For this review, take the finished solid that the model builds, in its own axes (mm). Give positions to 0.01 mm unless a question says otherwise; leave off trailing zeros. Order: outer loops, then holes, each group sorted by start corner. A loop starts at its lowest first (then second) coordinate and runs counter-clockwise, first axis right, second up. Notation, with made-up numbers: (1, 0.25) -> (31, 0.25) arc R22 ccw to (31, 31.25) -> close; hole circle Ø3 at (-28.5, 57). An arc over 180 degrees is marked (long way). Return JSON: item names as keys, results as strings. Group by question number.
1) To check wall thickness, follow line 1 along X through (y, z) = (61, 4.5); line 2 along X through (y, z) = (83.1, 0.9); line 3 along Z through (x, y) = (4.25, 79). State the ranges of each line that lie inside material, in increasing order.
2) Insertion check: P1, Ø5, axis at y = 66, z = 8.5, coming from the -X side; P2, Ø2.5, axis at x = 2, z = 4, coming from the +Y side; P3, Ø1.5, axis at x = 1.5, z = 6, coming from the +Y side. Each pin has a flat end and moves straight along its axis. Give the tip position at first contact, or say it passes through.
3) Add section D-D (y = 6). Give the boundary of the cut face in (x, z).
4) Add section A-A (y = -4.5). Give the boundary of the cut face in (x, z).
5) Add section B-B (z = 6). State how many separate pieces and enclosed holes the cut face has, then the cut area to 4 significant figures.
Autodesk Fusion 360 part; units mm, degrees
sketch "スケッチ1" plane through (0, 0, 0) normal (0, 0, 1) x (1, 0, 0)
  line L0 (1.5, 1.2) -> (3.5, 1.2)
  line L1 (3.5, 1.2) -> (3.5, 2.4)
  line L2 (3.5, 2.4) -> (1.5, 2.4)
  line L3 (1.5, 2.4) -> (1.5, 1.2)
  line L4 (1.5, 6.2) -> (3.5, 6.2)
  line L5 (3.5, 7.4) -> (1.5, 7.4)
  line L6 (3.5, 6.2) -> (3.5, 7.4)
  line L7 (1.5, 7.4) -> (1.5, 6.2)
  line L8 (1.5, 11.2) -> (3.5, 11.2)
  line L9 (3.5, 12.4) -> (1.5, 12.4)
  line L10 (3.5, 11.2) -> (3.5, 12.4)
  line L11 (1.5, 12.4) -> (1.5, 11.2)
  line L12 (1.5, 16.2) -> (3.5, 16.2)
  line L13 (3.5, 17.4) -> (1.5, 17.4)
  line L14 (3.5, 16.2) -> (3.5, 17.4)
  line L15 (1.5, 17.4) -> (1.5, 16.2)
  line L16 (1.5, 21.2) -> (3.5, 21.2)
  line L17 (3.5, 22.4) -> (1.5, 22.4)
  line L18 (3.5, 21.2) -> (3.5, 22.4)
  line L19 (1.5, 22.4) -> (1.5, 21.2)
  line L20 (1.5, 26.2) -> (3.5, 26.2)
  line L21 (3.5, 27.4) -> (1.5, 27.4)
  line L22 (3.5, 26.2) -> (3.5, 27.4)
  line L23 (1.5, 27.4) -> (1.5, 26.2)
  line L24 (1.5, 31.2) -> (3.5, 31.2)
  line L25 (3.5, 32.4) -> (1.5, 32.4)
  line L26 (3.5, 31.2) -> (3.5, 32.4)
  line L27 (1.5, 32.4) -> (1.5, 31.2)
  line L28 (1.5, 36.2) -> (3.5, 36.2)
  line L29 (3.5, 37.4) -> (1.5, 37.4)
  line L30 (3.5, 36.2) -> (3.5, 37.4)
  line L31 (1.5, 37.4) -> (1.5, 36.2)
  line L32 (1.5, 41.2) -> (3.5, 41.2)
  line L33 (3.5, 42.4) -> (1.5, 42.4)
  line L34 (3.5, 41.2) -> (3.5, 42.4)
  line L35 (1.5, 42.4) -> (1.5, 41.2)
  line L36 (1.5, 46.2) -> (3.5, 46.2)
  line L37 (3.5, 47.4) -> (1.5, 47.4)
  line L38 (3.5, 46.2) -> (3.5, 47.4)
  line L39 (1.5, 47.4) -> (1.5, 46.2)
  line L40 (1.5, 51.2) -> (3.5, 51.2)
  line L41 (3.5, 52.4) -> (1.5, 52.4)
  line L42 (3.5, 51.2) -> (3.5, 52.4)
  line L43 (1.5, 52.4) -> (1.5, 51.2)
  line L44 (1.5, 56.2) -> (3.5, 56.2)
  line L45 (3.5, 57.4) -> (1.5, 57.4)
  line L46 (3.5, 56.2) -> (3.5, 57.4)
  line L47 (1.5, 57.4) -> (1.5, 56.2)
  line L48 (1.5, 61.2) -> (3.5, 61.2)
  line L49 (3.5, 62.4) -> (1.5, 62.4)
  line L50 (3.5, 61.2) -> (3.5, 62.4)
  line L51 (1.5, 62.4) -> (1.5, 61.2)
  line L52 (1.5, 66.2) -> (3.5, 66.2)
  line L53 (3.5, 67.4) -> (1.5, 67.4)
  line L54 (3.5, 66.2) -> (3.5, 67.4)
  line L55 (1.5, 67.4) -> (1.5, 66.2)
  line L56 (1.5, 71.2) -> (3.5, 71.2)
  line L57 (3.5, 72.4) -> (1.5, 72.4)
  line L58 (3.5, 71.2) -> (3.5, 72.4)
  line L59 (1.5, 72.4) -> (1.5, 71.2)
  line L60 (1.5, 76.2) -> (3.5, 76.2)
  line L61 (3.5, 77.4) -> (1.5, 77.4)
  line L62 (3.5, 76.2) -> (3.5, 77.4)
  line L63 (1.5, 77.4) -> (1.5, 76.2)
  line L64 (0, 78.6) -> (5, 78.6)
  line L65 (5, 78.6) -> (5, 0)
  line L66 (5, 0) -> (0, 0)
  line L67 (0, 0) -> (0, 78.6)
  line L68 (6.5, -1.5) -> (-1.5, -1.5)
  line L69 (-1.5, -1.5) -> (-1.5, 80.1)
  line L70 (-1.5, 80.1) -> (6.5, 80.1)
  line L71 (6.5, 80.1) -> (6.5, -1.5)
  line L72 (0, 5.1) -> (5, 5.1)
  line L73 (5, 5.1) -> (5, 3.6)
  line L74 (5, 3.6) -> (0, 3.6)
  line L75 (0, 3.6) -> (0, 5.1)
  line L76 (5, 8.6) -> (0, 8.6)
  line L77 (0, 10.1) -> (5, 10.1)
  line L78 (5, 13.6) -> (0, 13.6)
  line L79 (0, 15.1) -> (5, 15.1)
  line L80 (5, 18.6) -> (0, 18.6)
  line L81 (0, 20.1) -> (5, 20.1)
  line L82 (5, 23.6) -> (0, 23.6)
  line L83 (0, 25.1) -> (5, 25.1)
  line L84 (5, 28.6) -> (0, 28.6)
  line L85 (0, 30.1) -> (5, 30.1)
  line L86 (5, 33.6) -> (0, 33.6)
  line L87 (0, 35.1) -> (5, 35.1)
  line L88 (5, 38.6) -> (0, 38.6)
  line L89 (0, 40.1) -> (5, 40.1)
  line L90 (5, 43.6) -> (0, 43.6)
  line L91 (0, 45.1) -> (5, 45.1)
  line L92 (5, 48.6) -> (0, 48.6)
  line L93 (0, 50.1) -> (5, 50.1)
  line L94 (5, 53.6) -> (0, 53.6)
  line L95 (0, 55.1) -> (5, 55.1)
  line L96 (5, 58.6) -> (0, 58.6)
  line L97 (0, 60.1) -> (5, 60.1)
  line L98 (5, 63.6) -> (0, 63.6)
  line L99 (0, 65.1) -> (5, 65.1)
  line L100 (5, 68.6) -> (0, 68.6)
  line L101 (0, 70.1) -> (5, 70.1)
  line L102 (5, 73.6) -> (0, 73.6)
  line L103 (0, 75.1) -> (5, 75.1)
  line L104 (-1.5, 80.1) -> (6.5, 80.1)
  line L105 (6.5, 80.1) -> (6.5, 86.1)
  line L106 (6.5, 86.1) -> (-1.5, 86.1)
  line L107 (-1.5, 86.1) -> (-1.5, 80.1)
  circle A0 centre (2.5, 83.1) radius 1.75
  line L108 (-1.5, -1.5) -> (6.5, -1.5)
  line L109 (6.5, -1.5) -> (6.5, -7.5)
  line L110 (6.5, -7.5) -> (-1.5, -7.5)
  line L111 (-1.5, -7.5) -> (-1.5, -1.5)
  circle A1 centre (2.5, -4.5) radius 1.75
  dimension "d1" = 2
  dimension "d2" = 1.2
  dimension "d5" = 0
  dimension "d6" = 75
  dimension "d7" = 78.6
  dimension "d8" = 1.2
  dimension "d9" = 5
  dimension "d10" = 1.5
  dimension "d11" = -1.5
  dimension "d12" = 1.5
  dimension "d15" = 0
  dimension "d16" = 70
  dimension "d17" = 1.2
  dimension "d18" = 8
  dimension "d19" = 6
  dimension "d20" = 3.5
  dimension "d21" = 4
  dimension "d22" = 3
  dimension "d23" = 8
  dimension "d24" = 6
  dimension "d25" = 3.5
  dimension "d26" = 4
  dimension "d27" = 3
extrude "押し出し1" add sketch "スケッチ1" along normal blind 5 contours L68 L69 L70 L71 L104 L108
extrude "押し出し2" add sketch "スケッチ1" along normal blind 9.5 contours L65 L67 L102 L103 | L65 L67 L100 L101 | L65 L67 L98 L99 | L65 L67 L96 L97 | L65 L67 L94 L95 | L65 L67 L92 L93 | L65 L67 L90 L91 | L65 L67 L88 L89 | L65 L67 L86 L87 | L65 L67 L84 L85 | L65 L67 L82 L83 | L65 L67 L80 L81 | L65 L67 L78 L79 | L65 L67 L76 L77 | L65 L67 L72 L73 L74 L75
extrude "押し出し3" add sketch "スケッチ1" along normal blind 2 contours L68 L108 L109 L110 L111 | L70 L104 L105 L106 L107
equation "d7 = 80 mm - 1.4 mm"
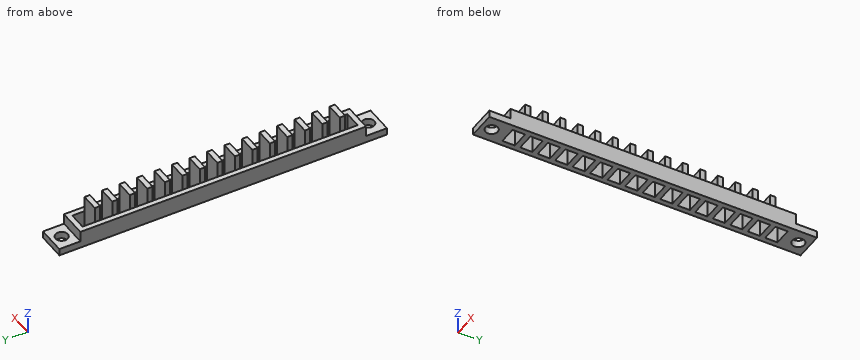
Evaluation:
{
 "1": {"line 1": "-1.5 to 0, 5 to 6.5", "line 2": "-1.5 to 0.75, 4.25 to 6.5", "line 3": "0 to 5"},
 "2": {"P1": "x = 0", "P2": "y = 80.1", "P3": "y = 75.1"},
 "3": {"outline": "(-1.5, 0) -> (0, 0) -> (0, 5) -> (-1.5, 5) -> close; (5, 0) -> (6.5, 0) -> (6.5, 5) -> (5, 5) -> close"},
 "4": {"outline": "(-1.5, 0) -> (0.75, 0) -> (0.75, 2) -> (-1.5, 2) -> close; (4.25, 0) -> (6.5, 0) -> (6.5, 2) -> (4.25, 2) -> close"},
 "5": {"separate pieces": "15", "enclosed holes": "0", "area": "112.5 mm^2"}
}
